Input: part model. Units: mm. Frame: model coordinates. A direction names the side the tool comes from. Coordinates: 2 decimals unless noted, no trailing zeros. Write each loop counter-clockwise with the first axis right and the second up, starting at its lowest first coordinate (ties: lowest second). Pieces come first, ordered by that corner, then holes. Notation, with made-up numbers: M 25.5,-11.5 L 48.5,-11.5 A22 ccw 48.5,-1.5 Z; hole C 86.25,70.5 d6. An arc over 180 degrees is marked long. Use one line per item in the form item = value.
from build123d import *

# Parameters (mm, degrees)
F0_W     = 122
F0_H     = 90
F0_W_2   = 56
F0_H_2   = 84
F0_W_3   = 54
F0_H_3   = 69
F1_DEPTH = 14
F2_DEPTH = 4
F3_DEPTH = 11
F4_R     = 5


with BuildPart() as f1:
    # F0 (on Front) → F1 (new body)
    with BuildSketch(Plane.XZ):
        with Locations((-16.471726, -0.079399)):
            Rectangle(F0_W, F0_H)
        with Locations((-46.471726, -0.079399)):
            Rectangle(F0_W_2, F0_H_2, mode=Mode.SUBTRACT)
        with Locations((14.528274, -0.079399)):
            Rectangle(F0_W_3, F0_H_3, mode=Mode.SUBTRACT)
    extrude(amount=F1_DEPTH)

    # F0 (on Front) → F2 (join)
    with BuildSketch(Plane.XZ):
        with Locations((-46.471726, -0.079399)):
            Rectangle(F0_W_2, F0_H_2)
    extrude(amount=F2_DEPTH)

    # F0 (on Front) → F3 (join)
    with BuildSketch(Plane.XZ):
        with Locations((14.528274, -0.079399)):
            Rectangle(F0_W_3, F0_H_3)
    extrude(amount=F3_DEPTH)

    # F4
    f4_edges = [f1.edges().sort_by_distance(p)[0] for p in [
        (-77.471726, -7, -45.079399),
        (44.528274, -7, -45.079399),
        (44.528274, -7, 44.920601),
        (-77.471726, -7, 44.920601),
    ]]
    fillet(f4_edges, radius=F4_R)


solid = f1.part
(1) Set-up query: faces 1 (the flat face through (-17, 0, 1)), 2 (the flat face through (-47, -9, -42.079)). Return all of +Z, -Z, +X, -X, +Y, -Y with unobstructed straight access to the full face (end or side cutting, diameter ignored); none if empty.
Computed:
face_1 = +Z, -Z, +X, -X, +Y
face_2 = -Y
(2) Section query D-D on x = 15. Return the cut outline in (y, z), plus the area to 3 significant figures.
Computed:
outline = M -14,-45.08 L 0,-45.08 L 0,44.92 L -14,44.92 L -14,34.42 L -11,34.42 L -11,-34.58 L -14,-34.58 Z
area = 1,050 mm^2
(3) Section query C-C on z = -1.5. Return the cut outline in (x, y), plus the area to 3 significant figures.
Computed:
outline = M -77.47,-14 L -74.47,-14 L -74.47,-4 L -18.47,-4 L -18.47,-14 L -12.47,-14 L -12.47,-11 L 41.53,-11 L 41.53,-14 L 44.53,-14 L 44.53,0 L -77.47,0 Z
area = 986 mm^2
(4) Section query B-B on x = -60.5. Return the cut outline in (y, z), plus the area to 3 significant figures.
Computed:
outline = M -14,-45.08 L 0,-45.08 L 0,44.92 L -14,44.92 L -14,41.92 L -4,41.92 L -4,-42.08 L -14,-42.08 Z
area = 420 mm^2
(5) Pull-direction query (Z, two-part tool) for faces 3 (the flat face through (-12.472, -12, -1)), 4 (the flat face through (-77.472, -7, -1)), 5 (the cylindrical face through (-76.046, -7.098, 43.417)); classes: pulls with the +Z half, pulls with the -Z half, needs draft (parallel to the pull), parting line crosses it, or undercut.
Computed:
face_3 = undercut
face_4 = needs draft
face_5 = pulls with the +Z half
(6) Section query A-A on y = -8.5. Return the cut outline in (x, z).
Computed:
outline = M -77.47,-40.08 A5 ccw -72.47,-45.08 L 39.53,-45.08 A5 ccw 44.53,-40.08 L 44.53,39.92 A5 ccw 39.53,44.92 L -72.47,44.92 A5 ccw -77.47,39.92 Z; hole M -74.47,-42.08 L -18.47,-42.08 L -18.47,41.92 L -74.47,41.92 Z
(7) Line query: probe 1 along X at (y, z) = (-12.25, -13); probe 2 along X at (y, z) = (-10.75, -34); probe 3 along Z at (x, y) = (-32.5, -9.5). Output: solid intervals per line, ascending.
Computed:
probe_1 = -77.47 to -74.47, -18.47 to -12.47, 41.53 to 44.53
probe_2 = -77.47 to -74.47, -18.47 to 44.53
probe_3 = -45.08 to -42.08, 41.92 to 44.92
